The drawing under review shows one solid part. Ordinate dimensions are in mm from its lowest x, y, z. A direction names the side the tool comes from. Coordinates: 2 decimals unless noted, no trailing zeros. Loops run counter-clockwise (first coordinate to the right, second up) from the corner with the lowest first, then second, coordinate; pieces in that order, holes last. Notation, with made-up numbers: (84.25, -36.5) -> (129.25, -36.5) arc R24 cw to (129.25, -12.5) -> close; hole circle Ø2 at (83, 61). An arc over 180 degrees is marked (long way). Use a Markdown table: item, result.
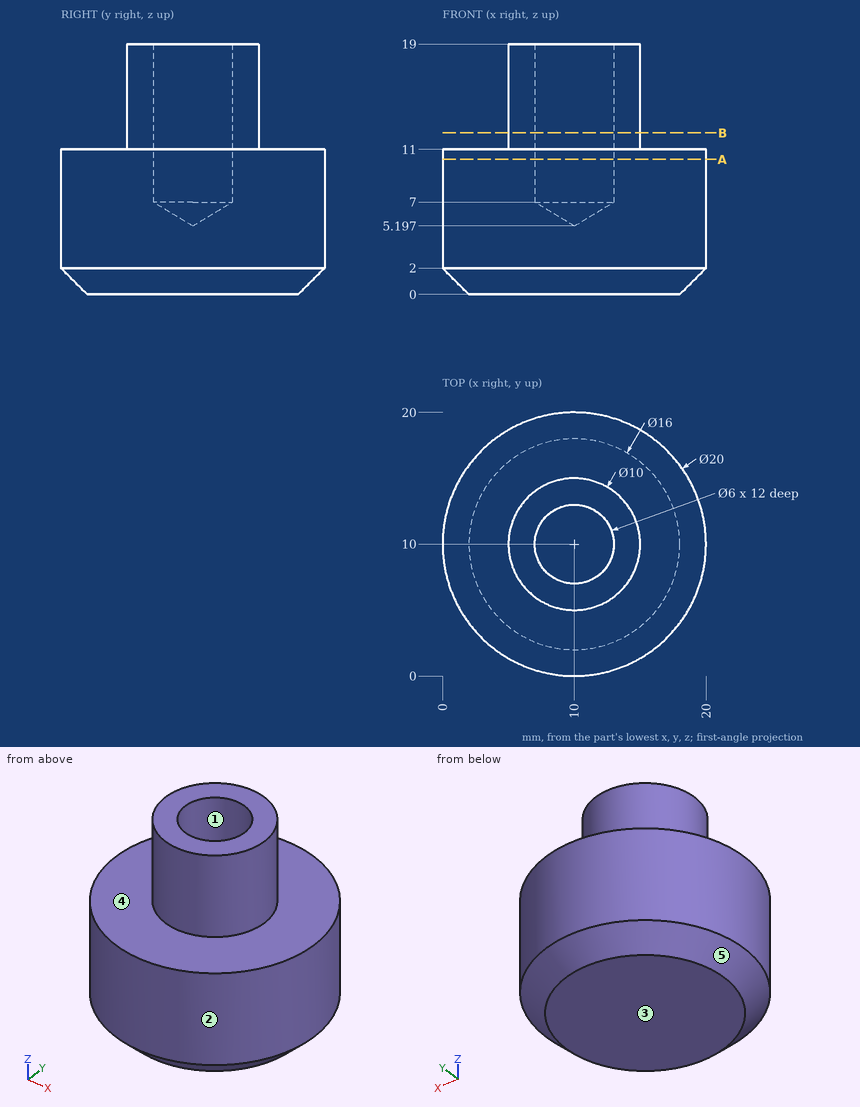
(1) Take a section at A-A on z = 10.25. Write out the cut boundary in (x, y), plus the area to 3 significant figures.
Found:
| item | result |
|---|---|
| outline | circle Ø20 at (10, 10); hole circle Ø6 at (10, 10) |
| area | 286 mm^2 |
(2) Take a section at B-B on z = 12.25. Write out the cut boundary in (x, y).
Found:
| item | result |
|---|---|
| outline | circle Ø10 at (10, 10); hole circle Ø6 at (10, 10) |
(3) For line 1 along Y through (x, z) = (10, 10.75); line 2 along Y through (x, z) = (10, 12); line 3 along X through (y, z) = (12.5, 12.25) (1 decimal), list the stretches that pass through material, from the lowest coordinate up.
Found:
| item | result |
|---|---|
| line 1 | y = 0 to 7, 13 to 20 |
| line 2 | y = 5 to 7, 13 to 15 |
| line 3 | x = 5.7 to 8.3, 11.7 to 14.3 |
(4) For the marked faces 4 and 5, list the 3-axis set-ups (+Z, -Z, +X, -X, +Y, -Y) from which the entire face can be reached by the end or side of a thin tool; tool diameter is ignored.
Found:
| item | result |
|---|---|
| face 4 | +Z |
| face 5 | -Z |
(5) For pin 1 Ø2 at (x, z) = (15.5, 13.5) entering from +Y; pin 2 Ø10 at (x, z) = (7.5, 16.5) entering from +Y; pin 3 Ø2 at (y, z) = (12, 4) entering from -X, all flat-tipped, find the tip position at first contact; note any pin that passes through.
Found:
| item | result |
|---|---|
| pin 1 | stops at y = 12.18 |
| pin 2 | stops at y = 15 |
| pin 3 | stops at x = 0.05 |
(6) Mouldability with a two-part tool opening along X and no side actions: class the marked faces 1, 2 and 3 as pulls with the +X half, pulls with the -X half, needs draft (parallel to the pull), parting line crosses it, or undercut.
Found:
| item | result |
|---|---|
| face 1 | undercut |
| face 2 | parting line crosses it |
| face 3 | needs draft |
